Part print with two shaded views. Sizes in mm from the minimum x, y, z corner. A direction names the side the tool comes from. Give positions to 0.01 mm unless a question says otherwise; leave off trailing zeros. Write each loop counter-clockwise with the first axis right and the second up, starting at its lowest first coordinate (ties: lowest second). Pieces come first, ordered by that corner, then holes. Notation, with made-up numbers: (89.5, 85) - (112.5, 85) arc R16 cw to (112.5, 109) - close; hole circle Ø4 at (-29, -30.5). An arc over 180 degrees is marked (long way). One line per item, written item: value. Start each with the question number.
(1) Cut at A-A, the plane z = 8.5. List the corners of the cut face in (x, y), and give its area (3 significant figures).
(2) 3-axis set-ups, long thin cutter, end or side, ignore diameter. For the marked faces 1, 2 and 3: which of +Z, -Z, +X, -X, +Y, -Y reach the whole face in a straight line?
(3) Cut at C-C, the plane x = 4. List the corners of the cut face in (y, z).
(4) Probe L1, parallel to Y at x = 28, z = 8; L2, parallel to Z at x = 26.5, y = 2.75; L3, parallel to X at y = 4.5, z = 14.25. List the from-to ranges inside material, lowest first.
(5) Cut at B-B, the plane y = 2.5. List the corners of the cut face in (x, z).
(6) Drop flat-ended pins along their axis: P1, Ø1.5, axis at x = 5.5, y = 2, coming from the -Z side; P2, Ø6, axis at x = 30, z = 7, coming from the -Y side; P3, Ø4.5, axis at x = 28, z = 7, coming from the +Y side; P4, Ø4, axis at x = 27, y = 3, coming from the +Z side. Give the stop position or say it passes through.
(7) Cut at D-D, the plane y = 6.25. List the corners of the cut face in (x, z), and give its area (3 significant figures).
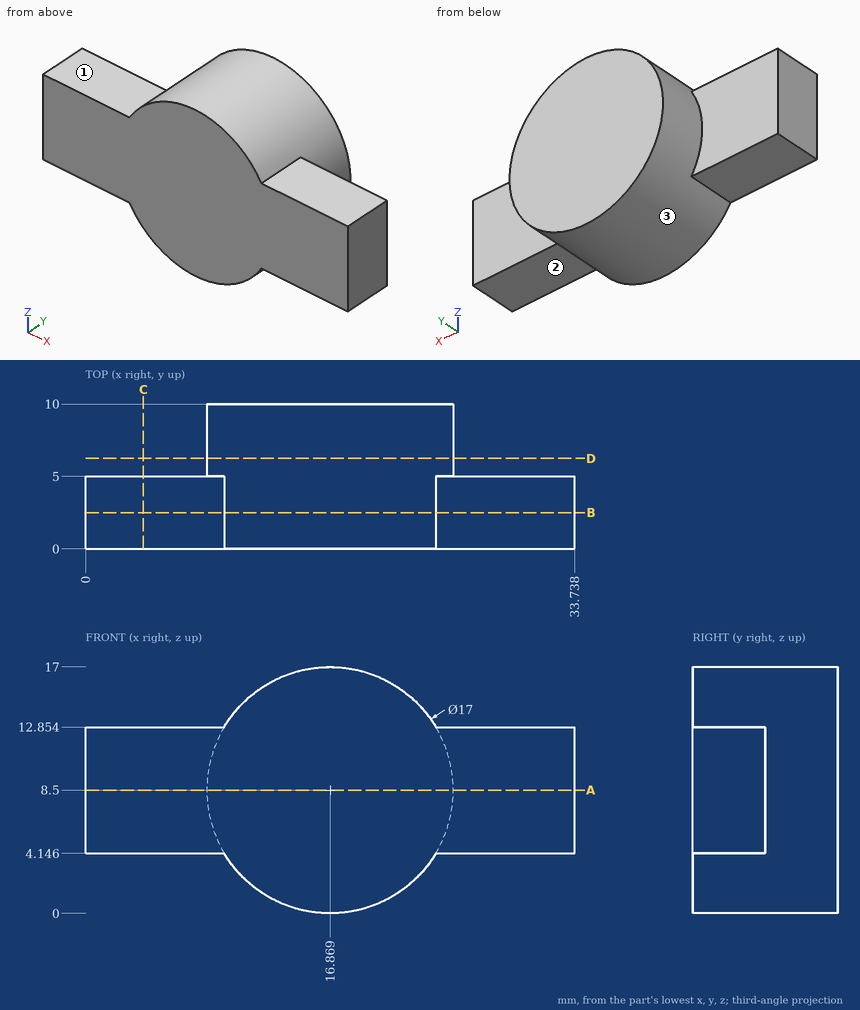
Answers follow:
1. outline: (0, 0) - (33.74, 0) - (33.74, 5) - (25.37, 5) - (25.37, 10) - (8.37, 10) - (8.37, 5) - (0, 5) - close
1. area: 254 mm²
2. face 1: +Z, -X, +Y, -Y
2. face 2: -Z, +X, +Y, -Y
2. face 3: +Y
3. outline: (0, 4.15) - (5, 4.15) - (5, 12.85) - (0, 12.85) - close
4. L1: y = 0 to 5
4. L2: z = 4.15 to 12.85
4. L3: x = 10.61 to 23.13
5. outline: (0, 4.15) - (9.57, 4.15) arc R8.5 ccw to (24.17, 4.15) - (33.74, 4.15) - (33.74, 12.85) - (24.17, 12.85) arc R8.5 ccw to (9.57, 12.85) - (0, 12.85) - close
6. P1: stops at z = 4.15
6. P2: stops at y = 0
6. P3: stops at y = 5
6. P4: stops at z = 12.85
7. outline: circle Ø17 at (16.87, 8.5)
7. area: 227 mm²
